```python
from build123d import *

# Parameters (mm, degrees)
SKETCH1_W                      = 101
SKETCH1_H                      = 10
SKETCH2_R                      = 79
BOSS_EXTRUDE1_DEPTH            = 35
F_8_4_8_4_DIAMETER_HOLE1_D     = 8.4
F_8_4_8_4_DIAMETER_HOLE1_DEPTH = 45
HOLE1_D                        = 120


with BuildPart() as part:
    # Sketch1 → Revolve1 (revolve)
    with BuildSketch(Plane(origin=(0, 0, 0), x_dir=(1, 0, 0), z_dir=(0, 1, 0))):
        with Locations((50.5, 5)):
            Rectangle(SKETCH1_W, SKETCH1_H)
    revolve(axis=Axis((0, 0, -10), (0, 0, 1)))

    # Sketch2 → Boss-Extrude1 (add)
    with BuildSketch(Plane.XY):
        Circle(SKETCH2_R)
    extrude(amount=BOSS_EXTRUDE1_DEPTH)

    # Sketch3 → Cut-Revolve1 (revolve, cut)
    with BuildSketch(Plane(origin=(0, 69.5, 0), x_dir=(1, 0, 0), z_dir=(0, 1, 0)), mode=Mode.PRIVATE) as cut_revolve1_sk:
        Polygon((3.3235, 10), (0, 10), (0, -5), (3.3235, -3.003039733), (3.3235, 0), align=None)
    revolve(cut_revolve1_sk.sketch.rotate(Axis((0, 69.5, -10), (0, 0, 1)), 180), axis=Axis((0, 69.5, -10), (0, 0, 1)), mode=Mode.SUBTRACT)

    # Sketch4 → Cut-Revolve2 (revolve, cut)
    with BuildSketch(Plane(origin=(0, 56.226681109, 0), x_dir=(1, 0, 0), z_dir=(0, 1, 0)), mode=Mode.PRIVATE) as cut_revolve2_sk:
        Polygon((44.174575034, 10), (40.851075034, 10), (40.851075034, -5), (44.174575034, -3.003039733), (44.174575034, 0), align=None)
    revolve(cut_revolve2_sk.sketch.rotate(Axis((40.851075034, 56.226681109, -10), (0, 0, 1)), 180), axis=Axis((40.851075034, 56.226681109, -10), (0, 0, 1)), mode=Mode.SUBTRACT)

    # Sketch5 → Cut-Revolve3 (revolve, cut)
    with BuildSketch(Plane(origin=(0, 21.476681109, 0), x_dir=(1, 0, 0), z_dir=(0, 1, 0)), mode=Mode.PRIVATE) as cut_revolve3_sk:
        Polygon((69.421927883, 10), (66.098427883, 10), (66.098427883, -5), (69.421927883, -3.003039733), (69.421927883, 0), align=None)
    revolve(cut_revolve3_sk.sketch.rotate(Axis((66.098427883, 21.476681109, -10), (0, 0, 1)), 180), axis=Axis((66.098427883, 21.476681109, -10), (0, 0, 1)), mode=Mode.SUBTRACT)

    # Sketch6 → Cut-Revolve4 (revolve, cut)
    with BuildSketch(Plane(origin=(0, -21.476681109, 0), x_dir=(1, 0, 0), z_dir=(0, 1, 0)), mode=Mode.PRIVATE) as cut_revolve4_sk:
        Polygon((69.421927883, 10), (66.098427883, 10), (66.098427883, -5), (69.421927883, -3.003039733), (69.421927883, 0), align=None)
    revolve(cut_revolve4_sk.sketch.rotate(Axis((66.098427883, -21.476681109, -10), (0, 0, 1)), 180), axis=Axis((66.098427883, -21.476681109, -10), (0, 0, 1)), mode=Mode.SUBTRACT)

    # Sketch7 → Cut-Revolve5 (revolve, cut)
    with BuildSketch(Plane(origin=(0, -56.226681109, 0), x_dir=(1, 0, 0), z_dir=(0, 1, 0)), mode=Mode.PRIVATE) as cut_revolve5_sk:
        Polygon((44.174575034, 10), (40.851075034, 10), (40.851075034, -5), (44.174575034, -3.003039733), (44.174575034, 0), align=None)
    revolve(cut_revolve5_sk.sketch.rotate(Axis((40.851075034, -56.226681109, -10), (0, 0, 1)), 180), axis=Axis((40.851075034, -56.226681109, -10), (0, 0, 1)), mode=Mode.SUBTRACT)

    # Sketch8 → Cut-Revolve6 (revolve, cut)
    with BuildSketch(Plane(origin=(0, -69.5, 0), x_dir=(1, 0, 0), z_dir=(0, 1, 0)), mode=Mode.PRIVATE) as cut_revolve6_sk:
        Polygon((3.3235, 10), (0, 10), (0, -5), (3.3235, -3.003039733), (3.3235, 0), align=None)
    revolve(cut_revolve6_sk.sketch.rotate(Axis((0, -69.5, -10), (0, 0, 1)), 180), axis=Axis((0, -69.5, -10), (0, 0, 1)), mode=Mode.SUBTRACT)

    # Sketch9 → Cut-Revolve7 (revolve, cut)
    with BuildSketch(Plane(origin=(0, -56.226681109, 0), x_dir=(1, 0, 0), z_dir=(0, 1, 0)), mode=Mode.PRIVATE) as cut_revolve7_sk:
        Polygon((-37.527575034, 10), (-40.851075034, 10), (-40.851075034, -5), (-37.527575034, -3.003039733), (-37.527575034, 0), align=None)
    revolve(cut_revolve7_sk.sketch.rotate(Axis((-40.851075034, -56.226681109, -10), (0, 0, 1)), 180), axis=Axis((-40.851075034, -56.226681109, -10), (0, 0, 1)), mode=Mode.SUBTRACT)

    # Sketch10 → Cut-Revolve8 (revolve, cut)
    with BuildSketch(Plane(origin=(0, -21.476681109, 0), x_dir=(1, 0, 0), z_dir=(0, 1, 0)), mode=Mode.PRIVATE) as cut_revolve8_sk:
        Polygon((-62.774927883, 10), (-66.098427883, 10), (-66.098427883, -5), (-62.774927883, -3.003039733), (-62.774927883, 0), align=None)
    revolve(cut_revolve8_sk.sketch.rotate(Axis((-66.098427883, -21.476681109, -10), (0, 0, 1)), 180), axis=Axis((-66.098427883, -21.476681109, -10), (0, 0, 1)), mode=Mode.SUBTRACT)

    # Sketch11 → Cut-Revolve9 (revolve, cut)
    with BuildSketch(Plane(origin=(0, 21.476681109, 0), x_dir=(1, 0, 0), z_dir=(0, 1, 0)), mode=Mode.PRIVATE) as cut_revolve9_sk:
        Polygon((-62.774927883, 10), (-66.098427883, 10), (-66.098427883, -5), (-62.774927883, -3.003039733), (-62.774927883, 0), align=None)
    revolve(cut_revolve9_sk.sketch.rotate(Axis((-66.098427883, 21.476681109, -10), (0, 0, 1)), 180), axis=Axis((-66.098427883, 21.476681109, -10), (0, 0, 1)), mode=Mode.SUBTRACT)

    # Sketch12 → Cut-Revolve10 (revolve, cut)
    with BuildSketch(Plane(origin=(0, 56.226681109, 0), x_dir=(1, 0, 0), z_dir=(0, 1, 0)), mode=Mode.PRIVATE) as cut_revolve10_sk:
        Polygon((-37.527575034, 10), (-40.851075034, 10), (-40.851075034, -5), (-37.527575034, -3.003039733), (-37.527575034, 0), align=None)
    revolve(cut_revolve10_sk.sketch.rotate(Axis((-40.851075034, 56.226681109, -10), (0, 0, 1)), 180), axis=Axis((-40.851075034, 56.226681109, -10), (0, 0, 1)), mode=Mode.SUBTRACT)

    # Ø8.4 (8.4) Diameter Hole1
    with Locations(Plane(origin=(0, 0, -10), x_dir=(-1, 0, 0), z_dir=(0, 0, -1))):
        with Locations((27.811529494, 85.595086467), (72.811529494, 52.900672706), (90, 0), (72.811529494, -52.900672706), (27.811529494, -85.595086467), (-27.811529494, -85.595086467), (-72.811529494, -52.900672706), (-90, 0), (-72.811529494, 52.900672706), (-27.811529494, 85.595086467)):
            Hole(F_8_4_8_4_DIAMETER_HOLE1_D / 2, depth=F_8_4_8_4_DIAMETER_HOLE1_DEPTH)

    # Hole1 (through all)
    with Locations(Plane(origin=(0, 0, -10), x_dir=(-1, 0, 0), z_dir=(0, 0, -1))):
        with Locations((0, 0)):
            Hole(HOLE1_D / 2)


solid = part.part
```
Could you check a few things on this model? Use its own coordinates, in mm. A direction names the side the tool comes from. Round coordinates to 2 decimals unless told otherwise and drop trailing zeros. Loops run counter-clockwise (first coordinate to the right, second up) from the corner with the lowest first, then second, coordinate; pieces in that order, holes last.
Q1. I want a section at B-B (x = 90). Write out the boundary of the cut face in (y, z), and give its area (3 significant figures).
Q2. On a 3-axis mill with a long thin cutter (end or side, diameter ignored), from which of +Z, -Z, +X, -X, +Y, -Y can I reach the whole of each face in a straight line? I mean faces 1 (the flat face through (30, -74, 0)), 2 (the cylindrical face through (-59.94, 2.64, 12.81)), 3 (the cylindrical face through (-1.79, 66.7, -3.59)). Say none if no direction works.
Q3. Please list where these lines run through material, in increasing order: L1, parallel to Y at x = -40.5, z = -7; L2, parallel to X at y = -47.5, z = 13; L3, parallel to Z at x = 76.5, y = -29.
Q4. I want a section at A-A (y = 0). Write out the boundary of the cut face in (x, z), and give its area (3 significant figures).
Q5. For P1, Ø6, axis at x = 66.1, y = -21.48, coming from the -Z side; P2, Ø12, axis at x = -40.5, z = 18.5, coming from the -Y side; P3, Ø1.5, axis at y = 69, z = 20.5, coming from the +X side; P4, Ø7.5, axis at x = -72.81, y = -52.9, coming from the -Z side, each with a flat end and sliding along its axis, tell me the tip position at first contact or that it passes through.
Q6. I want a section at C-C (y = -45). Write out the boundary of the cut face in (x, z).
Q7. Thinking about a two-plate mould opening in Y: for faces 4 (the flat face through (-12, 59, 35)), 5 (the cylindrical face through (93.88, -1.61, -4.93)), 6 (the conical face through (66.174, -22.049, 4.653)), which applies, pulls with the +Y half, pulls with the -Y half, needs draft (parallel to the pull), parting line crosses it, or undercut?
Q8. I want a section at D-D (z = 16). Write out the boundary of the cut face in (x, y).
Answer below:
1. outline: (-45.84, -10) - (-4.2, -10) - (-4.2, 0) - (-45.84, 0) - close; (4.2, -10) - (45.84, -10) - (45.84, 0) - (4.2, 0) - close
1. area: 833 mm2
2. face 1: +Z
2. face 2: +Z, -Z
2. face 3: -Z
3. L1: y = -92.52 to -59.53, -52.92 to -44.27, 44.27 to 52.92, 59.53 to 92.52
3. L2: x = -63.12 to -36.66, 36.66 to 63.12
3. L3: z = -10 to 0
4. outline: (-101, -10) - (-94.2, -10) - (-94.2, 0) - (-101, 0) - close; (-85.8, -10) - (-60, -10) - (-60, 35) - (-79, 35) - (-79, 0) - (-85.8, 0) - close; (60, -10) - (85.8, -10) - (85.8, 0) - (79, 0) - (79, 35) - (60, 35) - close; (94.2, -10) - (101, -10) - (101, 0) - (94.2, 0) - close
4. area: 1,980 mm2
5. P1: stops at z = 3.2
5. P2: stops at y = -71.07
5. P3: stops at x = 39.79
5. P4: passes through
6. outline: (-90.42, -10) - (-39.69, -10) - (-39.69, 35) - (-64.93, 35) - (-64.93, 0) - (-90.42, 0) - close; (39.69, -10) - (90.42, -10) - (90.42, 0) - (64.93, 0) - (64.93, 35) - (39.69, 35) - close
7. face 4: needs draft
7. face 5: undercut
7. face 6: undercut
8. outline: circle Ø158 at (0, 0); hole circle Ø120 at (0, 0)
